from build123d import *

# Parameters (mm, degrees)
SKETCH1_R           = 6.5
BOSS_EXTRUDE1_DEPTH = 20
SKETCH2_R           = 2
CUT_EXTRUDE1_DEPTH  = 7


with BuildPart() as part:
    # Sketch1 → Boss-Extrude1 (new body)
    with BuildSketch(Plane(origin=(0, 0, 0), x_dir=(1, 0, 0), z_dir=(0, 1, 0))):
        with Locations(Location((0, 0, 0), (0, 0, 270))):
            Circle(SKETCH1_R)
    extrude(amount=BOSS_EXTRUDE1_DEPTH)

    # Sketch2 → Cut-Extrude1 (cut)
    with BuildSketch(Plane.XZ):
        with Locations(Location((0, 0, 0), (0, 0, 270))):
            Circle(SKETCH2_R)
    extrude(amount=-CUT_EXTRUDE1_DEPTH, mode=Mode.SUBTRACT)

    # Sketch3 → Cut-Revolve1 (revolve, cut)
    with BuildSketch(Plane.XY):
        with BuildLine():
            Line((0, 30.9), (0, 17.9))
            ThreePointArc((0, 17.9), (-6.5, 24.4), (0, 30.9))
        make_face()
    revolve(axis=Axis((0, 20, 0), (0, -1, 0)), mode=Mode.SUBTRACT)


solid = part.part
Could you check a few things on this model? Use its own coordinates, in mm. A direction names the side the tool comes from. Coordinates: 2 decimals unless noted, no trailing zeros. Write each loop counter-clockwise with the first axis right and the second up, starting at its lowest first coordinate (ties: lowest second). Pieces come first, ordered by that corner, then holes. Notation, with made-up numbers: (57.5, 60.25) - (61.5, 60.25) arc R10 ccw to (61.5, 67.25) - close; hole circle Ø10 at (-10, 50). An arc over 180 degrees is marked (long way). Write item = value, one per line.
1) Suppose I cut it at D-D on y = 2.5. Please give me the cut outline in (x, z), plus the area to 3 significant figures.
Result set:
outline = circle Ø13 at (0, 0); hole circle Ø4 at (0, 0)
area = 120 mm2
2) For faces 4 (the flat face through (0, 7, 0)), 5 (the flat face through (2, 0, 1)), which set-ups out of +Z, -Z, +X, -X, +Y, -Y let a thin tool reach every point of the face, with its end or its side?
Result set:
face_4 = -Y
face_5 = +Z, -Z, +X, -X, -Y
3) We'd pull the mould along X, two halves only. Please class faces 1 (the cylindrical face through (-3.955, 9.86, -5.158)), 2 (the cylindrical face through (-2, 3, 0)), 3 (the flat face through (5, 20, -1)): +X half, -X half, draft (parallel to the pull), parting line (faces both ways), or undercut.
Result set:
face_1 = parting line
face_2 = undercut
face_3 = draft
4) Will these pins go through, and if not, where does the flat tip stop? pin 1 Ø4.5 at (x, z) = (0, 0) entering from +Y; pin 2 Ø1 at (x, z) = (1, -3) entering from +Y; pin 3 Ø4 at (y, z) = (10.5, 3.5) entering from -X.
Result set:
pin_1 = 18.3
pin_2 = 19.03
pin_3 = -6.32
5) Suppose I cut it at B-B on x = 0. Please give me the cut outline in (y, z).
Result set:
outline = (0, -6.5) - (20, -6.5) - (20, -4.78) arc R6.5 cw to (20, 4.78) - (20, 6.5) - (0, 6.5) - (0, 2) - (7, 2) - (7, -2) - (0, -2) - close
6) Please list where these lines run through material, in increasing order: line 1 (X direction, y = 2, z = 0); line 2 (Z direction, x = 0.25, y = 8.75); line 3 (X direction, y = 6, z = -1.75). Write a range as [from, to].
Result set:
line_1 = [-6.5, -2], [2, 6.5]
line_2 = [-6.5, 6.5]
line_3 = [-6.26, -0.97], [0.97, 6.26]
7) Suppose I cut it at A-A on z = 0. Please give me the cut outline in (x, y).
Result set:
outline = (-6.5, 0) - (-2, 0) - (-2, 7) - (2, 7) - (2, 0) - (6.5, 0) - (6.5, 20) - (4.78, 20) arc R6.5 cw to (-4.78, 20) - (-6.5, 20) - close
8) Suppose I cut it at C-C on y = 14. Please give me the cut outline in (x, z), plus the area to 3 significant figures.
Result set:
outline = circle Ø13 at (0, 0)
area = 133 mm2
